Check sheet for the modelled part. Datum: model origin and axes. Units: mm. A direction names the side the tool comes from. Round coordinates to 2 decimals unless told otherwise and drop trailing zeros. Order: outer loops, then holes, each group sorted by start corner. A loop starts at its lowest first (then second) coordinate and runs counter-clockwise, first axis right, second up. Notation, with made-up numbers: (-32.5, 25) -> (19.5, 25) arc R20 cw to (19.5, 32) -> close; hole circle Ø4 at (-27, -30.5). An arc over 180 degrees is marked (long way). Answer in a Markdown table with one row per item.
from build123d import *

# Parameters (mm, degrees)
SKETCH1_R           = 1.75
BOSS_EXTRUDE1_DEPTH = 0.5
SKETCH2_R           = 1.75
BOSS_EXTRUDE2_DEPTH = 1
BOSS_EXTRUDE3_START = -6
SKETCH3_R           = 3
SKETCH3_R_2         = 1.75
BOSS_EXTRUDE3_DEPTH = 6


with BuildPart() as part:
    # Sketch1 → Boss-Extrude1 (new, symmetric)
    with BuildSketch(Plane.XY):
        with BuildLine():
            Line((-4.261461708, 3.756090449), (-2.573402496, 2.862403135))
            ThreePointArc((-2.573402496, 2.862403135), (0, 2.223226069), (2.573402496, 2.862403135))
            Line((2.573402496, 2.862403135), (4.261461708, 3.756090449))
            ThreePointArc((4.261461708, 3.756090449), (10.5, 0), (4.261461708, -3.756090449))
            Line((4.261461708, -3.756090449), (2.573402496, -2.862403135))
            ThreePointArc((2.573402496, -2.862403135), (0, -2.223226069), (-2.573402496, -2.862403135))
            Line((-2.573402496, -2.862403135), (-4.261461708, -3.756090449))
            ThreePointArc((-4.261461708, -3.756090449), (-10.5, 0), (-4.261461708, 3.756090449))
        make_face()
        with Locations((-6.25, 0)):
            Circle(SKETCH1_R, mode=Mode.SUBTRACT)
        with Locations((6.25, 0)):
            Circle(SKETCH1_R, mode=Mode.SUBTRACT)
    extrude(amount=BOSS_EXTRUDE1_DEPTH, both=True)



with BuildPart() as body_2:
    # Sketch2 → Boss-Extrude2 (new body)
    with BuildSketch(Plane.XY.offset(5.5)):
        with BuildLine():
            Line((-2.573402496, 2.862403135), (-4.261461708, 3.756090449))
            ThreePointArc((-4.261461708, 3.756090449), (-10.5, 0), (-4.261461708, -3.756090449))
            Line((-4.261461708, -3.756090449), (-2.573402496, -2.862403135))
            ThreePointArc((-2.573402496, -2.862403135), (0, -2.223226069), (2.573402496, -2.862403135))
            Line((2.573402496, -2.862403135), (4.261461708, -3.756090449))
            ThreePointArc((4.261461708, -3.756090449), (10.5, 0), (4.261461708, 3.756090449))
            Line((4.261461708, 3.756090449), (2.573402496, 2.862403135))
            ThreePointArc((2.573402496, 2.862403135), (0, 2.223226069), (-2.573402496, 2.862403135))
        make_face()
        with Locations((6.25, 0)):
            Circle(SKETCH2_R, mode=Mode.SUBTRACT)
        with Locations((-6.25, 0)):
            Circle(SKETCH2_R, mode=Mode.SUBTRACT)
    extrude(amount=-BOSS_EXTRUDE2_DEPTH)


with BuildPart() as part_1:
    add(part.part)

    add(body_2.part)  # Boss-Extrude3 merges body 2
    # Sketch3 → Boss-Extrude3 (add)
    # profile 1 of 2: a face of its own
    with BuildSketch(Plane.XY.offset(5.5).offset(BOSS_EXTRUDE3_START)):
        with Locations((-6.25, 0)):
            Circle(SKETCH3_R)
        with Locations((-6.25, 0)):
            Circle(SKETCH3_R_2, mode=Mode.SUBTRACT)
    # profile 2 of 2: a face of its own
    with BuildSketch(Plane.XY.offset(5.5).offset(BOSS_EXTRUDE3_START)):
        with Locations((6.25, 0)):
            Circle(SKETCH3_R)
        with Locations((6.25, 0)):
            Circle(SKETCH3_R_2, mode=Mode.SUBTRACT)
    extrude(amount=BOSS_EXTRUDE3_DEPTH)


solid = part_1.part
Item 1: Cross-section at C-C (z = 4.7). Record the boundary of the cut face in (x, y).
Result sheet:
| item | result |
|---|---|
| outline | (-4.26, -3.76) -> (-2.57, -2.86) arc R5.5 cw to (2.57, -2.86) -> (4.26, -3.76) arc R4.25 ccw (long way) to (4.26, 3.76) -> (2.57, 2.86) arc R5.5 cw to (-2.57, 2.86) -> (-4.26, 3.76) arc R4.25 ccw (long way) to start; hole circle Ø3.5 at (-6.25, 0); hole circle Ø3.5 at (6.25, 0) |
Item 2: Cross-section at D-D (y = 2). Record the boundary of the cut face in (x, z).
Result sheet:
| item | result |
|---|---|
| outline | (-10, -0.5) -> (10, -0.5) -> (10, 0.5) -> (8.49, 0.5) -> (8.49, 4.5) -> (10, 4.5) -> (10, 5.5) -> (-10, 5.5) -> (-10, 4.5) -> (-8.49, 4.5) -> (-8.49, 0.5) -> (-10, 0.5) -> close; hole (-4.01, 0.5) -> (4.01, 0.5) -> (4.01, 4.5) -> (-4.01, 4.5) -> close |
Item 3: Cross-section at A-A (y = 0). Record the boundary of the cut face in (x, z).
Result sheet:
| item | result |
|---|---|
| outline | (-10.5, -0.5) -> (-8, -0.5) -> (-8, 5.5) -> (-10.5, 5.5) -> (-10.5, 4.5) -> (-9.25, 4.5) -> (-9.25, 0.5) -> (-10.5, 0.5) -> close; (-4.5, -0.5) -> (4.5, -0.5) -> (4.5, 5.5) -> (-4.5, 5.5) -> close; (8, -0.5) -> (10.5, -0.5) -> (10.5, 0.5) -> (9.25, 0.5) -> (9.25, 4.5) -> (10.5, 4.5) -> (10.5, 5.5) -> (8, 5.5) -> close; hole (-3.25, 0.5) -> (3.25, 0.5) -> (3.25, 4.5) -> (-3.25, 4.5) -> close |
Item 4: Cross-section at B-B (x = -6.25). Record the boundary of the cut face in (y, z), and give its area (3 significant figures).
Result sheet:
| item | result |
|---|---|
| outline | (-4.25, -0.5) -> (-1.75, -0.5) -> (-1.75, 5.5) -> (-4.25, 5.5) -> (-4.25, 4.5) -> (-3, 4.5) -> (-3, 0.5) -> (-4.25, 0.5) -> close; (1.75, -0.5) -> (4.25, -0.5) -> (4.25, 0.5) -> (3, 0.5) -> (3, 4.5) -> (4.25, 4.5) -> (4.25, 5.5) -> (1.75, 5.5) -> close |
| area | 20.0 mm^2 |
Item 5: Mould release check, pull along Z, two halves, no side actions. Record for faces 1 (the flat face through (0, 0, -0.5)), 2 (the cylindrical face through (-3.39, 0.9, 2.47)), 3 (the flat face through (-3.4, -3.3, 5)): pulls with the +Z half, pulls with the -Z half, needs draft (parallel to the pull), parting line crosses it, or undercut.
Result sheet:
| item | result |
|---|---|
| face 1 | pulls with the -Z half |
| face 2 | undercut |
| face 3 | needs draft |
Item 6: Depth check by flat-ended pin: P1, Ø3, axis at x = 6.25, y = 0, coming from the +Z side; P2, Ø1, axis at x = -5.5, z = 0.5, coming from the -Y side; P3, Ø1.5, axis at x = -4, z = 0.5, coming from the -Y side; P4, Ø3, axis at x = 2, z = 0.5, coming from the -Y side. Enter the tip coordinate at first touch or a pass-through.
Result sheet:
| item | result |
|---|---|
| P1 | passes through |
| P2 | stops at y = -4.24 |
| P3 | stops at y = -3.98 |
| P4 | stops at y = -3.35 |
Item 7: Set-up check for faces 4 (the flat face through (3.4, 3.3, 0)), 5 (the cylindrical face through (9.02, -1.15, 2.47)), 6 (the flat face through (3.4, -3.3, 0)), 7 (the cylindrical face through (10.5, -0.1, 5)): record each of +Z, -Z, +X, -X, +Y, -Y from which the full face is reachable in a straight line by a thin tool's end or side.
Result sheet:
| item | result |
|---|---|
| face 4 | +Z, -Z, +Y |
| face 5 | none |
| face 6 | +Z, -Z, -Y |
| face 7 | +Z, -Z |
Item 8: Scan lines: line 1 (Z direction, x = -2, y = 2); line 2 (Y direction, x = -6.25, z = 4.85); line 3 (Y direction, x = 6.25, z = 2.8). Record each from-to range of solid material in increasing order. Write a range as [from, to].
Result sheet:
| item | result |
|---|---|
| line 1 | z = [-0.5, 0.5], [4.5, 5.5] |
| line 2 | y = [-4.25, -1.75], [1.75, 4.25] |
| line 3 | y = [-3, -1.75], [1.75, 3] |
